from build123d import *

# Parameters (mm, degrees)
F0_W      = 152.4
F0_H      = 101.6
F1_DEPTH  = 3.175
F2_W      = 146.05
F2_H      = 3.175
F3_DEPTH  = 50.8
F5_DEPTH  = 25.4
F7_DEPTH  = 3.175
F8_DEPTH  = 25.4
F9_R      = 50.8
F10_DEPTH = 3.175
F11_R     = 50.8
F12_DEPTH = 3.175


# Not quite as in the source:
# - a length typed as a fraction of an inch, garbled in the dataset ("3 / 203.2 mm" for 3/8 in), is restored


with BuildPart() as f1:
    # F0 (on Top) → F1 (new body)
    with BuildSketch(Plane.XY):
        Rectangle(F0_W, F0_H)
    extrude(amount=F1_DEPTH)

    # F2 (on face) → F3 (join)
    with BuildSketch(Plane.XY.offset(3.175)):
        Polygon((-73.025, 50.8), (-76.2, 50.8), (-76.2, -50.8), (-73.025, -50.8), (-73.025, -47.625), (-73.025, 47.625), align=None)
        with Locations((0, 49.2125)):
            Rectangle(F2_W, F2_H)
        Polygon((76.2, 50.8), (73.025, 50.8), (73.025, 47.625), (73.025, -47.625), (73.025, -50.8), (76.2, -50.8), align=None)
        with Locations((0, -49.2125)):
            Rectangle(F2_W, F2_H)
    extrude(amount=F3_DEPTH)

    # F4 (on face) → F5 (cut)
    with BuildSketch(Plane.YZ.offset(76.2)):
        with BuildLine():
            ThreePointArc((1.5875, 26.9875), (0, 28.575), (-1.5875, 26.9875))
            Line((-1.5875, 26.9875), (1.5875, 26.9875))
        make_face()
        with BuildLine():
            Line((1.5875, 26.9875), (-1.5875, 26.9875))
            ThreePointArc((-1.5875, 26.9875), (0, 25.4), (1.5875, 26.9875))
        make_face()
    extrude(amount=-F5_DEPTH, mode=Mode.SUBTRACT)

    # F6 (on face) → F7 (cut)
    with BuildSketch(Plane(origin=(-76.2, 0, 0), x_dir=(0, -1, 0), z_dir=(-1, 0, 0))):
        with BuildLine():
            Line((-1.5875, 26.9875), (1.5875, 26.9875))
            ThreePointArc((1.5875, 26.9875), (0, 28.575), (-1.5875, 26.9875))
        make_face()
        with BuildLine():
            ThreePointArc((-1.5875, 26.9875), (0, 25.4), (1.5875, 26.9875))
            Line((1.5875, 26.9875), (-1.5875, 26.9875))
        make_face()
    extrude(amount=F7_DEPTH, mode=Mode.SUBTRACT)

    # F6 (on face) → F8 (cut)
    with BuildSketch(Plane(origin=(-76.2, 0, 0), x_dir=(0, -1, 0), z_dir=(-1, 0, 0))):
        with BuildLine():
            Line((-1.5875, 26.9875), (1.5875, 26.9875))
            ThreePointArc((1.5875, 26.9875), (0, 28.575), (-1.5875, 26.9875))
        make_face()
        with BuildLine():
            ThreePointArc((-1.5875, 26.9875), (0, 25.4), (1.5875, 26.9875))
            Line((1.5875, 26.9875), (-1.5875, 26.9875))
        make_face()
    extrude(amount=-F8_DEPTH, mode=Mode.SUBTRACT)

    # F9 (on face) → F10 (join)
    with BuildSketch(Plane.YZ.offset(76.2)):
        with Locations((0, 26.9875)):
            Circle(F9_R)
    extrude(amount=F10_DEPTH)

    # F11 (on face) → F12 (join)
    with BuildSketch(Plane(origin=(-76.2, 0, 0), x_dir=(0, -1, 0), z_dir=(-1, 0, 0))):
        with Locations((0, 26.9875)):
            Circle(F11_R)
    extrude(amount=F12_DEPTH)


solid = f1.part
Could you check a few things on this model? Use its own coordinates, in mm. A direction names the side the tool comes from. Give positions to 0.01 mm unless a question says otherwise; leave off trailing zeros. Order: outer loops, then holes, each group sorted by start corner. A loop starts at its lowest first (then second) coordinate and runs counter-clockwise, first axis right, second up.
1. Will these pins go through, and if not, where does the flat tip stop? P1, Ø8, axis at x = 63, y = -2.5, coming from the +Z side (3 decimals); P2, Ø1.5, axis at x = 44.5, y = 5, coming from the -Z side.
2. For faces 1 (the flat face through (76.2, -1, 63)), 2 (the flat face through (76.2, -1, -9)), 3 (the flat face through (73.025, 1, 23)), 4 (the cylindrical face through (-77.765, 6.613, 77.355)), 5 (the flat face through (76.2, 48, 48)), which set-ups out of +Z, -Z, +X, -X, +Y, -Y let a thin tool reach every point of the face, with its end or its side?
3. Suppose I cut it at C-C (z = 46). List the corners of the cut face in (x, y) for me (3 decimals), plus the area to 3 significant figures.
4. We'd pull the mould along X, two halves only. Please class faces 6 (the flat face through (-23, -49, 53.975)), 7 (the flat face through (76.2, -48, 6)), 8 (the flat face through (-76.2, -48, 6)): pulls with the +X half, pulls with the -X half, needs draft (parallel to the pull), parting line crosses it, or undercut.
5. Suppose I cut it at D-D (y = 5). List the corners of the cut face in (x, z) for me (3 decimals).
6. Suppose I cut it at B-B (x = -33). List the corners of the cut face in (y, z) for me (3 decimals), plus the area to 3 significant figures.
7. Suppose I cut it at A-A (z = -14). List the corners of the cut face in (x, y) for me (3 decimals), plus the area to 3 significant figures.
8. I need wall thicknesses on L1, parallel to X at y = 22.5, z = -4 (3 decimals); L2, parallel to Z at x = 74.1, y = 0 (3 decimals); L3, parallel to X at y = 6, z = 24 (3 decimals). Which ranges of each line are inside material? Lowest first, please.
Solved:
1. P1: stops at z = 3.175
1. P2: stops at z = 0
2. face 1: +Z, +Y, -Y
2. face 2: -Z, +Y, -Y
2. face 3: +Z
2. face 4: -X
2. face 5: +Z, +X, +Y
3. outline: (-79.375, -47.108) - (-76.2, -47.108) - (-76.2, -50.8) - (76.2, -50.8) - (76.2, -47.108) - (79.375, -47.108) - (79.375, 47.108) - (76.2, 47.108) - (76.2, 50.8) - (-76.2, 50.8) - (-76.2, 47.108) - (-79.375, 47.108) - close; hole (-73.025, -47.625) - (73.025, -47.625) - (73.025, 47.625) - (-73.025, 47.625) - close
3. area: 2,170 mm2
4. face 6: undercut
4. face 7: pulls with the +X half
4. face 8: pulls with the -X half
5. outline: (-79.375, -23.566) - (-76.2, -23.566) - (-76.2, 0) - (76.2, 0) - (76.2, -23.566) - (79.375, -23.566) - (79.375, 77.541) - (76.2, 77.541) - (76.2, 53.975) - (73.025, 53.975) - (73.025, 3.175) - (-73.025, 3.175) - (-73.025, 53.975) - (-76.2, 53.975) - (-76.2, 77.541) - (-79.375, 77.541) - close
6. outline: (-50.8, 0) - (50.8, 0) - (50.8, 53.975) - (47.625, 53.975) - (47.625, 3.175) - (-47.625, 3.175) - (-47.625, 53.975) - (-50.8, 53.975) - close
6. area: 645 mm2
7. outline: (-79.375, -30.011) - (-76.2, -30.011) - (-76.2, 30.011) - (-79.375, 30.011) - close; (76.2, -30.011) - (79.375, -30.011) - (79.375, 30.011) - (76.2, 30.011) - close
7. area: 381 mm2
8. L1: x = -79.375 to -76.2, 76.2 to 79.375
8. L2: z = 0 to 25.4, 28.575 to 53.975
8. L3: x = -79.375 to -73.025, 73.025 to 79.375
